Check sheet for the modelled part. Datum: model origin and axes. Units: mm. Give positions to 0.01 mm unless a question says otherwise; leave off trailing zeros. Order: outer loops, then holes, each group sorted by start corner. A loop starts at its lowest first (then second) coordinate and runs counter-clockwise, first axis right, second up.
Item 1: Sectioned sample at C-C on z = 0.9. Record the boundary of the cut face in (x, y) (3 decimals), and give its area (3 significant figures).
Item 2: Material ranges on line 1 along Y through (x, z) = (151.66, 1.05) (3 decimals); line 2 along Y through (x, z) = (89.08, 0.6) (3 decimals); line 3 along X through (y, z) = (-41, 2.7), recorded low to high.
Item 3: Sectioned sample at A-A on x = 26.5. Record the boundary of the cut face in (y, z) (3 decimals), and give its area (3 significant figures).
Item 4: Sectioned sample at B-B on y = -95. Record the boundary of the cut face in (x, z).
Item 5: Sectioned sample at D-D on y = -8. Record the boundary of the cut face in (x, z) (3 decimals).
Item 6: Gauge pin test, flat ends, axial feed: P1, Ø0.9, axis at x = 11.5, z = 1, coming from the -Y side; P2, Ø6.5, axis at x = 26.5, y = -110, coming from the -Z side. Record the tip position at first contact, or that the pin passes through.
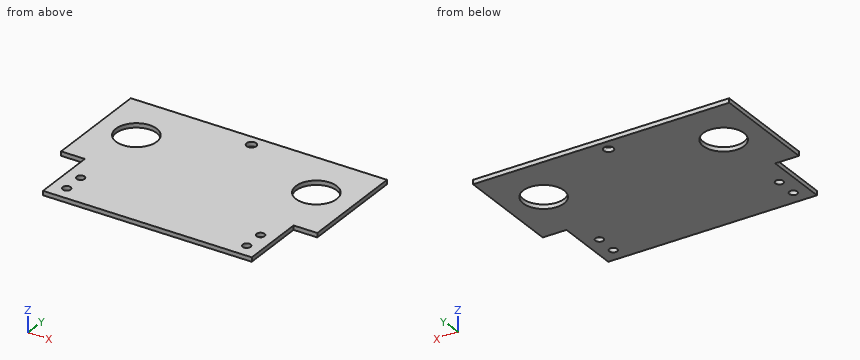
from build123d import *

# Parameters (mm, degrees)
SKETCH1_W           = 178.16
SKETCH1_H           = 120
BOSS_EXTRUDE1_DEPTH = 3
SKETCH2_R           = 14.225
SKETCH2_R_2         = 2.75
SKETCH2_R_3         = 3.375
CUT_EXTRUDE1_DEPTH  = 4
SKETCH3_W           = 16.5
SKETCH3_H           = 45
CUT_EXTRUDE2_DEPTH  = 4


with BuildPart() as part:
    # Sketch1 → Boss-Extrude1 (new body)
    with BuildSketch(Plane.XY):
        with Locations((89.08, -60)):
            Rectangle(SKETCH1_W, SKETCH1_H)
    extrude(amount=BOSS_EXTRUDE1_DEPTH)

    # Sketch2 → Cut-Extrude1 (cut, through all)
    with BuildSketch(Plane.XY.offset(3)):
        with Locations((26.5, -35)):
            Circle(SKETCH2_R)
        with Locations((151.66, -35)):
            Circle(SKETCH2_R)
        with Locations((26.5, -110)):
            Circle(SKETCH2_R_2)
        with Locations((151.66, -110)):
            Circle(SKETCH2_R_2)
        with Locations((89.08, -8)):
            Circle(SKETCH2_R_3)
        with Locations((26.5, -95)):
            Circle(SKETCH2_R_2)
        with Locations((151.66, -95)):
            Circle(SKETCH2_R_2)
    extrude(amount=-CUT_EXTRUDE1_DEPTH, mode=Mode.SUBTRACT)

    # Sketch3 → Cut-Extrude2 (cut, through all)
    with BuildSketch(Plane(origin=(0, 0, 0), x_dir=(-1, 0, 0), z_dir=(0, 0, -1))):
        with Locations((-8.25, -97.5)):
            Rectangle(SKETCH3_W, SKETCH3_H)
        with Locations((-169.91, -97.5)):
            Rectangle(SKETCH3_W, SKETCH3_H)
    extrude(amount=-CUT_EXTRUDE2_DEPTH, mode=Mode.SUBTRACT)


solid = part.part
Report:
1. outline: (0, -75) - (16.5, -75) - (16.5, -120) - (161.66, -120) - (161.66, -75) - (178.16, -75) - (178.16, 0) - (0, 0) - close; hole circle Ø28.45 at (26.5, -35); hole circle Ø5.5 at (26.5, -110); hole circle Ø5.5 at (26.5, -95); hole circle Ø6.75 at (89.08, -8); hole circle Ø28.45 at (151.66, -35); hole circle Ø5.5 at (151.66, -110); hole circle Ø5.5 at (151.66, -95)
1. area: 18,500 mm2
2. line 1: y = -120 to -112.75, -107.25 to -97.75, -92.25 to -49.225, -20.775 to 0
2. line 2: y = -120 to -11.375, -4.625 to 0
2. line 3: x = 0 to 13.6, 39.4 to 138.76, 164.56 to 178.16
3. outline: (-120, 0) - (-112.75, 0) - (-112.75, 3) - (-120, 3) - close; (-107.25, 0) - (-97.75, 0) - (-97.75, 3) - (-107.25, 3) - close; (-92.25, 0) - (-49.225, 0) - (-49.225, 3) - (-92.25, 3) - close; (-20.775, 0) - (0, 0) - (0, 3) - (-20.775, 3) - close
3. area: 242 mm2
4. outline: (16.5, 0) - (23.75, 0) - (23.75, 3) - (16.5, 3) - close; (29.25, 0) - (148.91, 0) - (148.91, 3) - (29.25, 3) - close; (154.41, 0) - (161.66, 0) - (161.66, 3) - (154.41, 3) - close
5. outline: (0, 0) - (85.705, 0) - (85.705, 3) - (0, 3) - close; (92.455, 0) - (178.16, 0) - (178.16, 3) - (92.455, 3) - close
6. P1: stops at y = -75
6. P2: stops at z = 0
